Check sheet for the modelled part. Datum: model origin and axes. Units: mm. Round coordinates to 2 decimals unless told otherwise and drop trailing zeros. Order: outer loops, then holes, each group sorted by start corner. A loop starts at its lowest first (then second) coordinate and runs counter-clockwise, first axis right, second up.
```python
from build123d import *

# Parameters (mm, degrees)
SKETCH1_R          = 29.25
EXTRUDE_3_8_DEPTH  = 9.525
CUT_EXTRUDE1_DEPTH = 9.525
SKETCH3_R          = 2.25
M4_THROUGH_DEPTH   = 9.525
SKETCH4_R          = 3.81
F_3_8_DRILL_DEPTH  = 9.525
SKETCH6_W          = 18.02935576
SKETCH6_H          = 57.579918791
CUT_EXTRUDE2_DEPTH = 9.525


with BuildPart() as part:
    # Sketch1 → 3/8 (new body)
    with BuildSketch(Plane.XY):
        with Locations(Location((0, 0, 0), (0, 0, 180))):
            Circle(SKETCH1_R)
    extrude(amount=EXTRUDE_3_8_DEPTH)

    # Sketch2 → Cut-Extrude1 (cut)
    with BuildSketch(Plane.XY.offset(9.525)):
        with BuildLine():
            Line((-3, 24.219267124), (-3, 18.154700472))
            ThreePointArc((-3, 18.154700472), (-3.409072822, 16.942697702), (-4.468950714, 16.226492325))
            ThreePointArc((-4.468950714, 16.226492325), (-5.859541661, 15.777716729), (-7.205966503, 15.210017108))
            ThreePointArc((-7.205966503, 15.210017108), (-9.131700947, 15.327380042), (-10.062257748, 17.017436623))
            Line((-10.062257748, 17.017436623), (-10.062257748, 23.378898605))
            ThreePointArc((-10.062257748, 23.378898605), (-9.690760884, 24.539922954), (-8.714280211, 25.269630397))
            ThreePointArc((-8.714280211, 25.269630397), (-7.073918129, 25.776977757), (-5.404367165, 26.177962402))
            ThreePointArc((-5.404367165, 26.177962402), (-3.736816389, 25.769869318), (-3, 24.219267124))
        make_face()
        with BuildLine():
            Line((-3, 10.72213294), (-3, 7.483314774))
            ThreePointArc((-3, 7.483314774), (-3.236165793, 6.540505732), (-3.888888889, 5.820355935))
            ThreePointArc((-3.888888889, 5.820355935), (-5.257283867, 4.621792546), (-6.270644915, 3.111111111))
            ThreePointArc((-6.270644915, 3.111111111), (-8.518752181, 2.052793582), (-10.062257748, 4))
            Line((-10.062257748, 4), (-10.062257748, 8.658183111))
            ThreePointArc((-10.062257748, 8.658183111), (-9.896091132, 9.45634044), (-9.425202627, 10.121870666))
            ThreePointArc((-9.425202627, 10.121870666), (-7.729958395, 11.468847089), (-5.845262531, 12.534736386))
            ThreePointArc((-5.845262531, 12.534736386), (-3.925412885, 12.408923541), (-3, 10.72213294))
        make_face()
        with BuildLine():
            Line((3, 10.72213294), (3, 7.483314774))
            ThreePointArc((3, 7.483314774), (3.236165793, 6.540505732), (3.888888889, 5.820355935))
            ThreePointArc((3.888888889, 5.820355935), (5.257283867, 4.621792546), (6.270644915, 3.111111111))
            ThreePointArc((6.270644915, 3.111111111), (8.518752181, 2.052793582), (10.062257748, 4))
            Line((10.062257748, 4), (10.062257748, 8.658183111))
            ThreePointArc((10.062257748, 8.658183111), (9.896091132, 9.45634044), (9.425202627, 10.121870666))
            ThreePointArc((9.425202627, 10.121870666), (7.729958395, 11.468847089), (5.845262531, 12.534736386))
            ThreePointArc((5.845262531, 12.534736386), (3.925412885, 12.408923541), (3, 10.72213294))
        make_face()
        with BuildLine():
            Line((3, 24.219267124), (3, 18.154700472))
            ThreePointArc((3, 18.154700472), (3.409072822, 16.942697702), (4.468950714, 16.226492325))
            ThreePointArc((4.468950714, 16.226492325), (5.859541661, 15.777716729), (7.205966503, 15.210017108))
            ThreePointArc((7.205966503, 15.210017108), (9.131700947, 15.327380042), (10.062257748, 17.017436623))
            Line((10.062257748, 17.017436623), (10.062257748, 23.378898605))
            ThreePointArc((10.062257748, 23.378898605), (9.690760884, 24.539922954), (8.714280211, 25.269630397))
            ThreePointArc((8.714280211, 25.269630397), (7.073918129, 25.776977757), (5.404367165, 26.177962402))
            ThreePointArc((5.404367165, 26.177962402), (3.736816389, 25.769869318), (3, 24.219267124))
        make_face()
        with BuildLine():
            Line((-3, -10.72213294), (-3, -7.483314774))
            ThreePointArc((-3, -7.483314774), (-3.236165793, -6.540505732), (-3.888888889, -5.820355935))
            ThreePointArc((-3.888888889, -5.820355935), (-5.257283867, -4.621792546), (-6.270644915, -3.111111111))
            ThreePointArc((-6.270644915, -3.111111111), (-8.518752181, -2.052793582), (-10.062257748, -4))
            Line((-10.062257748, -4), (-10.062257748, -8.658183111))
            ThreePointArc((-10.062257748, -8.658183111), (-9.896091132, -9.45634044), (-9.425202627, -10.121870666))
            ThreePointArc((-9.425202627, -10.121870666), (-7.729958395, -11.468847089), (-5.845262531, -12.534736386))
            ThreePointArc((-5.845262531, -12.534736386), (-3.925412885, -12.408923541), (-3, -10.72213294))
        make_face()
        with BuildLine():
            Line((3, -10.72213294), (3, -7.483314774))
            ThreePointArc((3, -7.483314774), (3.236165793, -6.540505732), (3.888888889, -5.820355935))
            ThreePointArc((3.888888889, -5.820355935), (5.257283867, -4.621792546), (6.270644915, -3.111111111))
            ThreePointArc((6.270644915, -3.111111111), (8.518752181, -2.052793582), (10.062257748, -4))
            Line((10.062257748, -4), (10.062257748, -8.658183111))
            ThreePointArc((10.062257748, -8.658183111), (9.896091132, -9.45634044), (9.425202627, -10.121870666))
            ThreePointArc((9.425202627, -10.121870666), (7.729958395, -11.468847089), (5.845262531, -12.534736386))
            ThreePointArc((5.845262531, -12.534736386), (3.925412885, -12.408923541), (3, -10.72213294))
        make_face()
        with BuildLine():
            Line((3, -24.219267124), (3, -18.154700472))
            ThreePointArc((3, -18.154700472), (3.409072822, -16.942697702), (4.468950714, -16.226492325))
            ThreePointArc((4.468950714, -16.226492325), (5.859541661, -15.777716729), (7.205966503, -15.210017108))
            ThreePointArc((7.205966503, -15.210017108), (9.131700947, -15.327380042), (10.062257748, -17.017436623))
            Line((10.062257748, -17.017436623), (10.062257748, -23.378898605))
            ThreePointArc((10.062257748, -23.378898605), (9.690760884, -24.539922954), (8.714280211, -25.269630397))
            ThreePointArc((8.714280211, -25.269630397), (7.073918129, -25.776977757), (5.404367165, -26.177962402))
            ThreePointArc((5.404367165, -26.177962402), (3.736816389, -25.769869318), (3, -24.219267124))
        make_face()
        with BuildLine():
            Line((-3, -24.219267124), (-3, -18.154700472))
            ThreePointArc((-3, -18.154700472), (-3.409072822, -16.942697702), (-4.468950714, -16.226492325))
            ThreePointArc((-4.468950714, -16.226492325), (-5.859541661, -15.777716729), (-7.205966503, -15.210017108))
            ThreePointArc((-7.205966503, -15.210017108), (-9.131700947, -15.327380042), (-10.062257748, -17.017436623))
            Line((-10.062257748, -17.017436623), (-10.062257748, -23.378898605))
            ThreePointArc((-10.062257748, -23.378898605), (-9.690760884, -24.539922954), (-8.714280211, -25.269630397))
            ThreePointArc((-8.714280211, -25.269630397), (-7.073918129, -25.776977757), (-5.404367165, -26.177962402))
            ThreePointArc((-5.404367165, -26.177962402), (-3.736816389, -25.769869318), (-3, -24.219267124))
        make_face()
    extrude(amount=-CUT_EXTRUDE1_DEPTH, mode=Mode.SUBTRACT)

    # Sketch3 → M4_through (cut)
    with BuildSketch(Plane.XY.offset(9.525)):
        with Locations((0, 15)):
            Circle(SKETCH3_R)
        with Locations((0, -15)):
            Circle(SKETCH3_R)
    extrude(amount=-M4_THROUGH_DEPTH, mode=Mode.SUBTRACT)

    # Sketch4 → 3/8_DRILL (cut)
    with BuildSketch(Plane.XY.offset(9.525)):
        Circle(SKETCH4_R)
    extrude(amount=-F_3_8_DRILL_DEPTH, mode=Mode.SUBTRACT)

    # Sketch6 → Cut-Extrude2 (cut)
    with BuildSketch(Plane.XY.offset(9.525)):
        with Locations((-22.076935628, -1.336167669)):
            Rectangle(SKETCH6_W, SKETCH6_H)
        with Locations((22.076935628, -1.336167669)):
            Rectangle(SKETCH6_W, SKETCH6_H)
    extrude(amount=-CUT_EXTRUDE2_DEPTH, mode=Mode.SUBTRACT)


solid = part.part
```
Item 1: Release check for a two-part mould opening along X. For faces 1 (the cylindrical face through (-0.488, 12.804, 4.829)), 2 (the flat face through (13.062, 0, 5)), 3 (the cylindrical face through (0.19, 29.25, 4.7)), 4 (the flat face through (3, -9, 5)) record: released by +X, released by -X, zero draft, split by the parting line, or undercut.
Answer:
face 1: undercut
face 2: released by +X
face 3: split by the parting line
face 4: undercut
Item 2: Sectioned sample at B-B (y = 0). Record the cut outline in (x, z) (3 decimals), and give its area (3 significant figures).
Answer:
outline: (-13.062, 0) - (-3.81, 0) - (-3.81, 9.525) - (-13.062, 9.525) - close; (3.81, 0) - (13.062, 0) - (13.062, 9.525) - (3.81, 9.525) - close
area: 176 mm2
Item 3: Sectioned sample at C-C (z = 7). State how many separate pieces and enclosed holes the cut face has, and give its area (3 significant figures).
Answer:
separate pieces: 1
enclosed holes: 11
area: 895 mm2
Item 4: Sectioned sample at A-A (x = 0). Record the cut outline in (y, z) (3 decimals), and give its area (3 significant figures).
Answer:
outline: (-29.25, 0) - (-17.25, 0) - (-17.25, 9.525) - (-29.25, 9.525) - close; (-12.75, 0) - (-3.81, 0) - (-3.81, 9.525) - (-12.75, 9.525) - close; (3.81, 0) - (12.75, 0) - (12.75, 9.525) - (3.81, 9.525) - close; (17.25, 0) - (29.25, 0) - (29.25, 9.525) - (17.25, 9.525) - close
area: 399 mm2
Item 5: Scan lines: line 1 along Y through (x, z) = (0, 6.5); line 2 along X through (y, z) = (-25, 7); line 3 along X through (y, z) = (17, 1.5). Record each from-to range of solid material in increasing order.
Answer:
line 1: y = -29.25 to -17.25, -12.75 to -3.81, 3.81 to 12.75, 17.25 to 29.25
line 2: x = -13.06 to -9.23, -3.16 to 3.16, 9.23 to 13.06
line 3: x = -13.06 to -10.06, -3.37 to -1.03, 1.03 to 3.37, 10.06 to 13.06
Item 6: Go/stop test with a flat-tipped pin: P1, Ø4, axis at x = 0, y = 15, coming from the -Z side. Record where the tip stops, or that it passes through.
Answer:
P1: passes through
